Read the model definition and answer for the solid it produces. Units are mm, in the model's axes. Face numbers are marked on the shaded views. A direction names the side the tool comes from. Round coordinates to 2 decimals unless told otherwise and drop trailing zeros. Loops run counter-clockwise (first coordinate to the right, second up) from the corner with the lowest first, then second, coordinate; pieces in that order, holes last. Notation, with made-up numbers: (-34, 39) - (15, 39) arc R21 ccw to (15, 73) - close; hole circle Ø3 at (4.5, -10.5). An arc over 180 degrees is marked (long way). Answer as CSV lines item,"result".
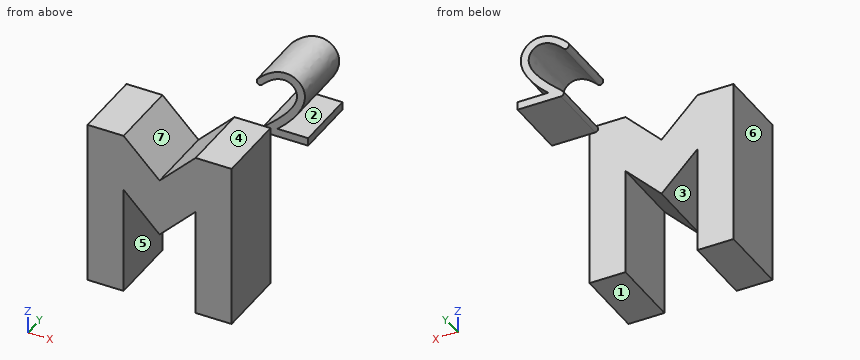
```python
from build123d import *

# Parameters (mm, degrees)
F1_DEPTH = 12.7
F3_DEPTH = 11.20158
F4_R     = 0.508


with BuildPart() as f1:
    # F0 (on Front) → F1 (new body)
    with BuildSketch(Plane.XZ):
        Polygon((-25.4, 29.21), (-25.4, 0), (-19.05, 0), (-19.05, 19.05), (-12.7, 12.7), (-6.35, 19.05), (-6.35, 0), (0, 0), (0, 29.21), (-6.35, 29.21), (-12.7, 22.86), (-19.05, 29.21), align=None)
    extrude(amount=F1_DEPTH)

    # F2 (on Front) → F3 (join)
    with BuildSketch(Plane.XZ):
        with BuildLine():
            Line((-2.3994161721, 28.0597675592), (6.6355378367, 28.0597675592))
            Line((6.6355378367, 28.0597675592), (6.6355378367, 29.4827252309))
            Line((6.6355378367, 29.4827252309), (1.2384620469, 29.4827252309))
            add(Edge.make_bspline(
                [(1.2384620469, 29.4827252309), (4.3676832704, 32.1977850174), (8.890126837, 38.6554285203), (1.7391745932, 42.078929022), (-2.3994161721, 37.6041723206)],
                knots=[0, 0, 0, 0, 0.5203529604, 1, 1, 1, 1], degree=3))
            Line((-2.3994161721, 37.6041723206), (-2.3994161721, 35.8844103642))
            add(Edge.make_bspline(
                [(-2.3994161721, 28.0597675592), (2.1288901598, 31.8470776853), (7.5727786172, 37.3091404259), (1.4697099185, 40.5985963112), (-2.3994161721, 35.8844103642)],
                knots=[0, 0, 0, 0, 0.5601329519, 1, 1, 1, 1], degree=3))
        make_face()
    extrude(amount=-F3_DEPTH)

    # F4
    f4_edges = [f1.edges().sort_by_distance(p)[0] for p in [
        (-2.399416, 5.60079, 28.059768),
        (-2.399416, 5.60079, 35.88441),
    ]]
    fillet(f4_edges, radius=F4_R)


solid = f1.part
```
1) The mould has two halves that part along X. Classify the marked faces 4, 5, 6 and 7: pulls with the +X half, pulls with the -X half, needs draft (parallel to the pull), parting line crosses it, or undercut.
Entries:
face 4,"needs draft"
face 5,"undercut"
face 6,"pulls with the -X half"
face 7,"undercut"
2) Each of these flat-tipped pins is pushed along its axis until it touches: P1, Ø6.5, axis at y = -9.5, z = 6, coming from the +X side; P2, Ø7.5, axis at x = -11.5, z = 10.5, coming from the +Y side; P3, Ø12, axis at x = -6, z = 36, coming from the -Y side; P4, Ø6, axis at x = 3, y = 7, coming from the +Z side. Where does it stop, or does it pass through?
Entries:
P1,"stops at x = 0"
P2,"stops at y = 0"
P3,"stops at y = 0"
P4,"stops at z = 40.42"
3) A cutting plane is placed at A-A, the plane z = 26. Determine the outline of the cut face in (x, y).
Entries:
outline,"(-25.4, -12.7) - (-15.84, -12.7) - (-15.84, 0) - (-25.4, 0) - close; (-9.56, -12.7) - (0, -12.7) - (0, 0) - (-9.56, 0) - close"
4) A cutting plane is placed at B-B, the plane z = 15.5. Determine the outline of the cut face in (x, y), plus the area to 3 significant figures.
Entries:
outline,"(-25.4, -12.7) - (-19.05, -12.7) - (-19.05, 0) - (-25.4, 0) - close; (-15.5, -12.7) - (-9.9, -12.7) - (-9.9, 0) - (-15.5, 0) - close; (-6.35, -12.7) - (0, -12.7) - (0, 0) - (-6.35, 0) - close"
area,"232 mm^2"
5) A cutting plane is placed at D-D, the plane z = 7.5. Determine the outline of the cut face in (x, y).
Entries:
outline,"(-25.4, -12.7) - (-19.05, -12.7) - (-19.05, 0) - (-25.4, 0) - close; (-6.35, -12.7) - (0, -12.7) - (0, 0) - (-6.35, 0) - close"
6) A cutting plane is placed at C-C, the plane y = -10. Determine the outline of the cut face in (x, z), plus the area to 3 significant figures.
Entries:
outline,"(-25.4, 0) - (-19.05, 0) - (-19.05, 19.05) - (-12.7, 12.7) - (-6.35, 19.05) - (-6.35, 0) - (0, 0) - (0, 29.21) - (-6.35, 29.21) - (-12.7, 22.86) - (-19.05, 29.21) - (-25.4, 29.21) - close"
area,"500 mm^2"
7) A tool of negligible diameter and unlimited length cuts with its end or side. For the marked faces 1, 2 and 3, from which of +Z, -Z, +X, -X, +Y, -Y can it reach the whole face along a straight path? Write none if from no direction.
Entries:
face 1,"-Z, +X, -X, +Y, -Y"
face 2,"+X, +Y, -Y"
face 3,"-Z, +Y, -Y"
8) Find the intervals of material crossed by line 1 (X direction, y = -1.75, z = 14); line 2 (Z direction, x = 1.5, y = 6); line 3 (X direction, y = -9.5, z = 16), in increasing order.
Entries:
line 1,"x = -25.4 to -19.05, -14 to -11.4, -6.35 to 0"
line 2,"z = 28.06 to 29.48, 29.71 to 31.55, 38.92 to 40.26"
line 3,"x = -25.4 to -19.05, -16 to -9.4, -6.35 to 0"
